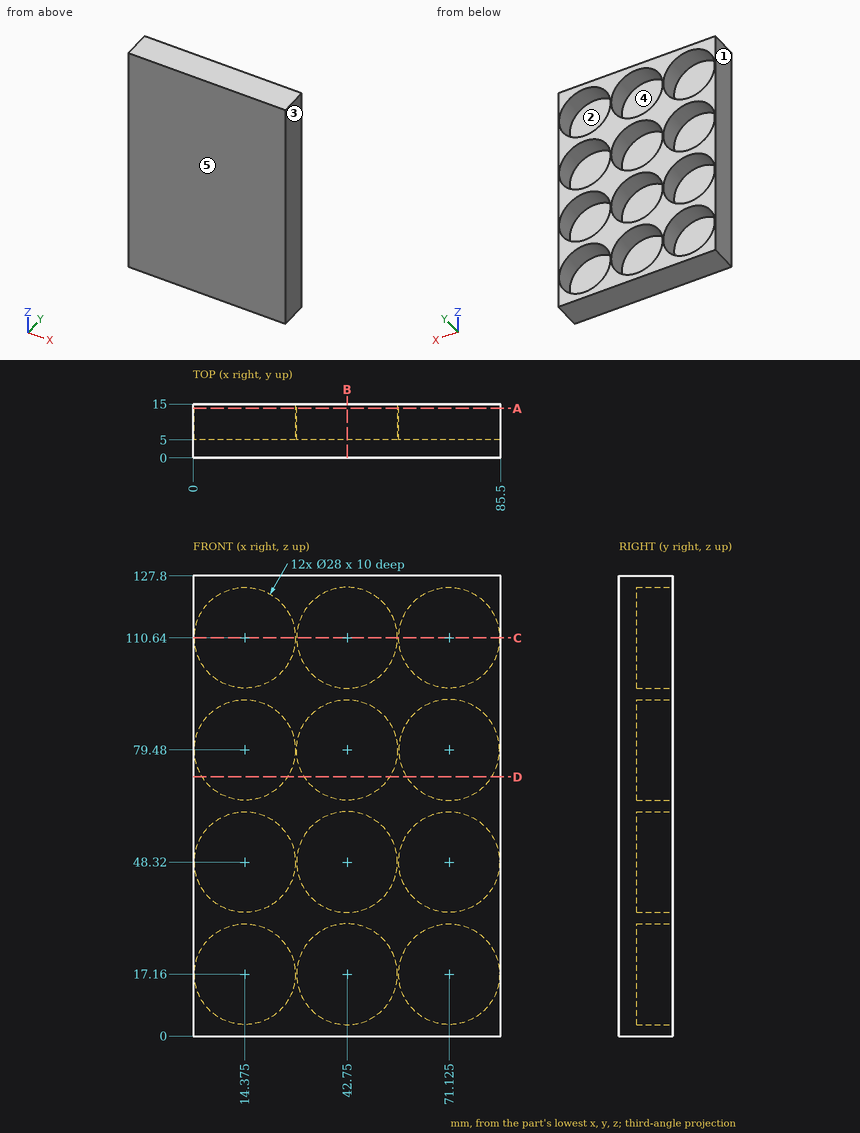
Check sheet for the drawn part. Datum: minimum x, y, z corner. Units: mm. A direction names the side the tool comes from. Give positions to 0.01 mm unless a question says otherwise; leave off trailing zeros. Loops run counter-clockwise (first coordinate to the right, second up) from the corner with the lowest first, then second, coordinate; pieces in that order, holes last.
1) Sectioned sample at C-C, the plane z = 110.64. Enter the section's corners in (x, y) (3 decimals).
2) Sectioned sample at B-B, the plane x = 42.75. Enter the section's corners in (y, z), then the cut area to 3 significant figures.
3) Sectioned sample at D-D, the plane z = 72. Enter the section's corners in (x, y), then the cut area to 3 significant figures.
4) Set-up check for the marked faces 1 and 2: record each of +Z, -Z, +X, -X, +Y, -Y from which the full face is reachable in a straight line by a thin tool's end or side.
5) Draft check along X on the marked faces 3, 4 and 5. Enter one of: pulls with the +X half, pulls with the -X half, needs draft (parallel to the pull), parting line crosses it, or undercut.
6) Thickness scan on line 1 along X through (y, z) = (9.5, 79.48) (3 decimals); line 2 along Z through (x, y) = (42.75, 8); line 3 along Z through (x, y) = (17, 12.5). Record the ranges inside material, lowest first.
7) Depth check by flat-ended pin: pin 1 Ø8.5 at (x, z) = (68, 106) entering from +Y. Enter the tip coordinate at first touch or a pass-through.
8) Sectioned sample at A-A, the plane y = 13.75. Count the separate pieces of the cut face and the enclosed holes in it, then the cut area to 3 significant figures.
Answers:
1. outline: (0, 0) - (85.5, 0) - (85.5, 15) - (85.125, 15) - (85.125, 5) - (57.125, 5) - (57.125, 15) - (56.75, 15) - (56.75, 5) - (28.75, 5) - (28.75, 15) - (28.375, 15) - (28.375, 5) - (0.375, 5) - (0.375, 15) - (0, 15) - close
2. outline: (0, 0) - (15, 0) - (15, 3.16) - (5, 3.16) - (5, 31.16) - (15, 31.16) - (15, 34.32) - (5, 34.32) - (5, 62.32) - (15, 62.32) - (15, 65.48) - (5, 65.48) - (5, 93.48) - (15, 93.48) - (15, 96.64) - (5, 96.64) - (5, 124.64) - (15, 124.64) - (15, 127.8) - (0, 127.8) - close
2. area: 797 mm2
3. outline: (0, 0) - (85.5, 0) - (85.5, 15) - (82.96, 15) - (82.96, 5) - (59.29, 5) - (59.29, 15) - (54.58, 15) - (54.58, 5) - (30.92, 5) - (30.92, 15) - (26.21, 15) - (26.21, 5) - (2.54, 5) - (2.54, 15) - (0, 15) - close
3. area: 572 mm2
4. face 1: +Z, -Z, -X, +Y, -Y
4. face 2: +Y
5. face 3: pulls with the +X half
5. face 4: undercut
5. face 5: needs draft
6. line 1: x = 0 to 0.375, 28.375 to 28.75, 56.75 to 57.125, 85.125 to 85.5
6. line 2: z = 0 to 3.16, 31.16 to 34.32, 62.32 to 65.48, 93.48 to 96.64, 124.64 to 127.8
6. line 3: z = 0 to 3.41, 30.91 to 34.57, 62.07 to 65.73, 93.23 to 96.89, 124.39 to 127.8
7. pin 1: stops at y = 5
8. separate pieces: 1
8. enclosed holes: 12
8. area: 3,540 mm2
